Here's the drawing with two shaded views (mm, measured from the low corner). I have some questions. Give positions to 0.01 mm unless a question says otherwise; leave off trailing zeros. Loops run counter-clockwise (first coordinate to the right, second up) from the corner with the lowest first, then second, coordinate; pieces in that order, holes last. Notation, with made-up numbers: M 42,8.25 L 63,8.25 A33 ccw 63,42.25 Z; hole C 20.5,-30 d5. An arc over 180 degrees is marked long. Put each result on its own line as item: value. Start each with the question number.
1) Please list where these lines run through material, in increasing order: line 1 along Y through (x, z) = (10, 6); line 2 along Z through (x, y) = (10.25, 3); line 3 along Y through (x, z) = (9, 8). Write a range as from..to.
2) Imagine slicing it at A-A (x = 10). Write out the boundary of the cut face in (y, z), then the cut area to 3 significant figures.
3) For P1, Ø1, axis at y = 11, z = 7.5, coming from the +X side; P2, Ø1, axis at y = 13.5, z = 2.5, coming from the +X side; P3, Ø5, axis at x = 6.5, y = 7, coming from the -Z side; P4, Ø5, axis at y = 18, z = 10, coming from the +X side, each with a flat end and sliding along its axis, tell me the tip position at first contact or that it passes through.
4) Imagine slicing it at C-C (z = 4). Write out the boundary of the cut face in (x, y), then the cut area to 3 significant figures.
5) If we mould it in two halves opening along Y, with no side actions, what happens to the marked faces 1, 2 and 3? For each: +Y half, -Y half, draft (parallel to the pull), parting line (faces both ways), or undercut.
6) Imagine slicing it at D-D (y = 13.75). Write out the boundary of the cut face in (x, z).
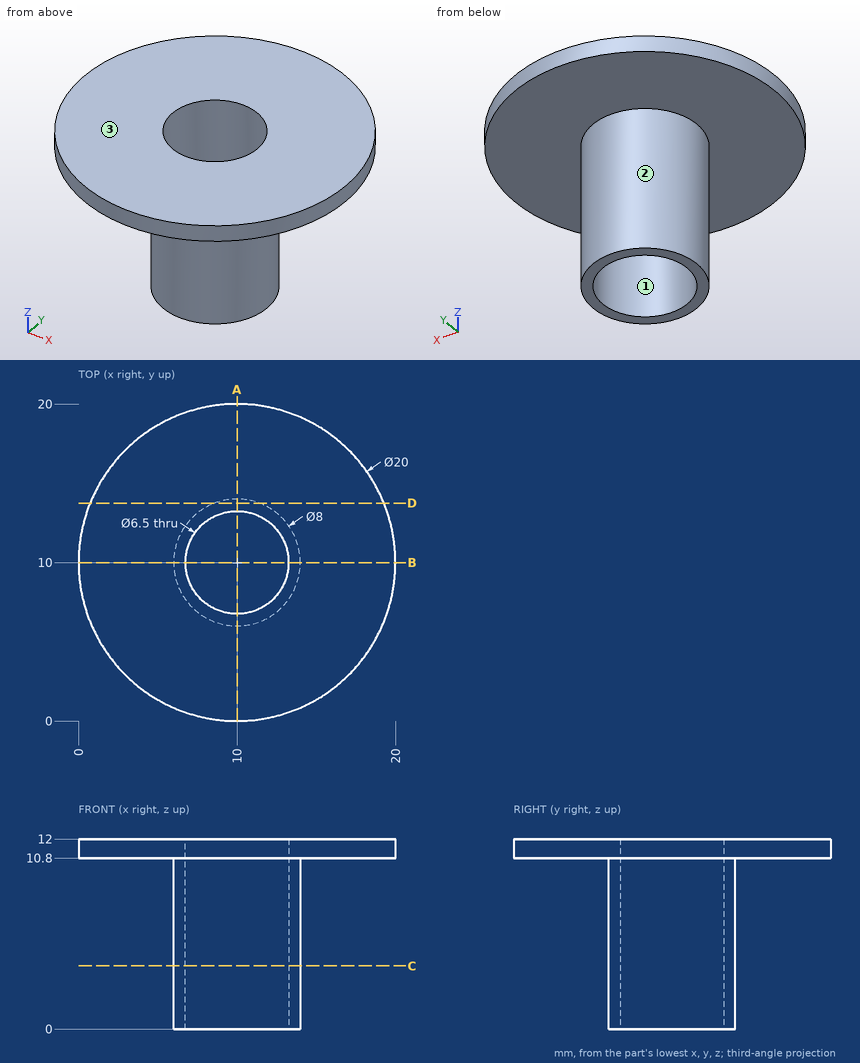
Recorded:
1. line 1: 6..6.75, 13.25..14
1. line 2: 10.8..12
1. line 3: 6.13..6.91, 13.09..13.87
2. outline: M 0,10.8 L 6,10.8 L 6,0 L 6.75,0 L 6.75,12 L 0,12 Z; M 13.25,0 L 14,0 L 14,10.8 L 20,10.8 L 20,12 L 13.25,12 Z
2. area: 32.4 mm²
3. P1: x = 13.97
3. P2: x = 12.65
3. P3: z = 0
3. P4: x = 18.26
4. outline: C 10,10 d8; hole C 10,10 d6.5
4. area: 17.1 mm²
5. face 1: undercut
5. face 2: parting line
5. face 3: draft
6. outline: M 0.73,10.8 L 8.61,10.8 L 8.61,0 L 11.39,0 L 11.39,10.8 L 19.27,10.8 L 19.27,12 L 0.73,12 Z
